```python
from build123d import *

# Parameters (mm, degrees)
F0_W     = 177.8
F0_H     = 127
F1_DEPTH = 3.175
F3_DEPTH = 3.175
F5_DEPTH = 3.175


with BuildPart() as f1:
    # F0 (on Front) → F1 (new body)
    with BuildSketch(Plane.XZ):
        Rectangle(F0_W, F0_H)
    extrude(amount=-F1_DEPTH)

    # F2 (on face) → F3 (cut, through all)
    with BuildSketch(Plane.XZ):
        Polygon((-38.1, -50.8), (-38.1, -57.15), (-2.54, -57.15), (-2.54, -50.8), (-7.62, -50.8), (-33.02, -50.8), align=None)
        Polygon((-33.02, 25.162934), (-33.02, -50.8), (-7.62, -50.8), (-7.62, 12.629322), (8.708571, 25.146), (8.708571, 57.15), align=None)
        Polygon((2.54, -57.15), (38.1, -57.15), (38.1, -50.8), (33.02, -50.8), (7.62, -50.8), (2.54, -50.8), align=None)
        Polygon((7.62, -50.8), (33.02, -50.8), (33.02, -4.329412), (40.47873, 1.388083), (40.47873, 33.392083), (7.62, 8.2042), align=None)
    extrude(amount=-F3_DEPTH, mode=Mode.SUBTRACT)

    # F4 (on face) → F5 (cut, through all)
    with BuildSketch(Plane.XZ):
        Polygon((-77.47, -14.746419), (-77.47, -31.75), (-77.47, -48.753581), (-70.485, -57.15), (-63.5, -57.15), (-63.5, -52.07), (-68.103037, -52.07), (-72.39, -46.916795), (-72.39, -31.75), (-72.39, -16.583205), (-68.103037, -11.43), (-63.5, -11.43), (-63.5, -6.35), (-70.485, -6.35), align=None)
        Polygon((-44.45, -14.746419), (-51.435, -6.35), (-58.42, -6.35), (-58.42, -11.43), (-53.816963, -11.43), (-49.53, -16.583205), (-49.53, -19.826419), (-44.45, -19.826419), align=None)
        Polygon((-58.42, -57.15), (-51.435, -57.15), (-44.45, -48.753581), (-44.45, -43.673581), (-49.53, -43.673581), (-49.53, -46.916795), (-53.816963, -52.07), (-58.42, -52.07), align=None)
        Polygon((58.547, -6.35), (44.45, -6.35), (44.45, -11.811), (46.99, -11.811), (46.99, -31.75), (46.99, -51.689), (44.45, -51.689), (44.45, -57.15), (58.547, -57.15), (58.547, -52.07), (52.07, -52.07), (52.07, -35.478037), (57.912, -35.478037), (57.912, -28.021963), (52.07, -28.021963), (52.07, -11.43), (58.547, -11.43), align=None)
        Polygon((77.47, -12.002101), (72.359407, -6.35), (63.627, -6.35), (63.627, -11.43), (70.104, -11.43), (72.39, -13.95822), (72.39, -25.424098), (68.834, -28.021963), (62.992, -28.021963), (62.992, -35.478037), (68.834, -35.478037), (72.39, -38.075902), (72.39, -49.54178), (70.104, -52.07), (63.627, -52.07), (63.627, -57.15), (72.359407, -57.15), (77.47, -51.497899), (77.47, -35.495899), (72.342551, -31.75), (77.47, -28.004101), align=None)
    extrude(amount=-F5_DEPTH, mode=Mode.SUBTRACT)


solid = f1.part
```
Model file for the job. Use its own axes, mm. A direction names the side the tool comes from. Coordinates: 2 decimals unless noted, no trailing zeros. Loops run counter-clockwise (first coordinate to the right, second up) from the corner with the lowest first, then second, coordinate; pieces in that order, holes last. Notation, with made-up numbers: (-1, -30) - (55, -30) arc R25 cw to (55, -8) - close; hole circle Ø3 at (22, -10.5). An arc over 180 degrees is marked (long way). Answer as a JSON object with one key per item and string values. Group by question number.
(1) Tool access for faces 1 (the face through (-51.643, 1.565, -49.457)), 2 (the face through (-1, 3.175, 1)): list every direction of +Z, -Z, +X, -X, +Y, -Y with a clear straight run to the whole face (end or side of a thin tool).
(2) Cut at C-C (x = -22). Give the cut face in (y, z) (3 decimals).
(3) Probe line 1 along Z through (x, y) = (54.5, 1.5); line 2 along X through (y, z) = (2.25, -23.5); line 3 along Z through (x, y) = (-56, 2.45). List the from-to ranges inside material, lowest first.
(4) Cut at A-A (z = 5). Give the cut face in (x, y) (3 decimals).
(5) Two-plate mould, pull along Z, no slides. Class faces 3 (the face through (-47.9, 1.6, -10.6)), 4 (the face through (-1, 0, 1)): released by +Z, released by -Z, zero draft, split by the parting line, or undercut.
(6) Flat gauge pins, fed straight in: pin 1 (1.5 mm diameter, centred on x = 50, z = -20, fed in from +Y); pin 2 (8 mm diameter, centred on x = -70, z = -1.5, fed in from -Y). Where does each tip first touch, or does it go through?
(7) Cut at D-D (y = 2.4). State how many separate pieces and enclosed holes the cut face has, then the cut area to 3 significant figures.
(8) Cut at B-B (z = 37.5). Give the cut face in (x, y) (3 decimals), then the cut area to 3 significant figures.
Geometry says:
{
 "1": {"face 1": "+Y, -Y", "face 2": "+Z, -Z, +X, -X, +Y"},
 "2": {"outline": "(0, -63.5) - (3.175, -63.5) - (3.175, -57.15) - (0, -57.15) - close; (0, 33.61) - (3.175, 33.61) - (3.175, 63.5) - (0, 63.5) - close"},
 "3": {"line 1": "z = -63.5 to -57.15, -52.07 to -35.48, -28.02 to -11.43, -6.35 to 63.5", "line 2": "x = -88.9 to -77.47, -72.39 to -33.02, -7.62 to 7.62, 33.02 to 46.99, 52.07 to 72.39, 77.47 to 88.9", "line 3": "z = -63.5 to -57.15, -52.07 to -11.43, -6.35 to 63.5"},
 "4": {"outline": "(-88.9, 0) - (-33.02, 0) - (-33.02, 3.175) - (-88.9, 3.175) - close; (-7.62, 0) - (7.62, 0) - (7.62, 3.175) - (-7.62, 3.175) - close; (40.479, 0) - (88.9, 0) - (88.9, 3.175) - (40.479, 3.175) - close"},
 "5": {"face 3": "undercut", "face 4": "zero draft"},
 "6": {"pin 1": "passes through", "pin 2": "stops at y = 0"},
 "7": {"separate pieces": "1", "enclosed holes": "7", "area": "16,200 mm^2"},
 "8": {"outline": "(-88.9, 0) - (-16.926, 0) - (-16.926, 3.175) - (-88.9, 3.175) - close; (8.709, 0) - (88.9, 0) - (88.9, 3.175) - (8.709, 3.175) - close", "area": "483 mm^2"}
}
